from build123d import *

# Parameters (mm, degrees)
EXTRUDE_1_DEPTH     = 10
EXTRUDE_2_DEPTH     = 10
SKETCH_4_W          = 32
SKETCH_4_H          = 4
EXTRUDE_3_DEPTH     = 60
CUT_EXTRUDE_1_DEPTH = 30
SKETCH_6_W          = 12
SKETCH_6_H          = 10
EXTRUDE_4_DEPTH     = 40
SKETCH_7_W          = 10
SKETCH_7_H          = 5
EXTRUDE_5_DEPTH     = 100
SKETCH_9_R          = 5
EXTRUDE_7_DEPTH     = 5


with BuildPart() as part:
    # 草图1 → 凸台-拉伸1 (new body)
    with BuildSketch(Plane(origin=(0, 0, 0), x_dir=(1, 0, 0), z_dir=(0, 1, 0))):
        with BuildLine():
            Line((-50, 0), (-46, 0))
            ThreePointArc((-46, 0), (0, 46), (46, 0))
            Line((46, 0), (50, 0))
            ThreePointArc((50, 0), (0, 50), (-50, 0))
        make_face()
    extrude(amount=EXTRUDE_1_DEPTH)

    # 草图3 → 凸台-拉伸2 (add)
    with BuildSketch(Plane(origin=(0, 10, 0), x_dir=(1, 0, 0), z_dir=(0, 1, 0))):
        with BuildLine():
            Line((-50, 16), (-47.370877129, 16))
            ThreePointArc((-47.370877129, 16), (-36.689752119, 33.968545589), (-19.595917942, 46))
            Line((-19.595917942, 46), (-30, 46))
            Line((-30, 46), (-30, 50))
            Line((-30, 50), (30, 50))
            Line((30, 50), (30, 46))
            Line((30, 46), (19.595917942, 46))
            ThreePointArc((19.595917942, 46), (36.689752119, 33.968545589), (47.370877129, 16))
            Line((47.370877129, 16), (50, 16))
            Line((50, 16), (50, -16))
            Line((50, -16), (46, -16))
            Line((46, -16), (46, 0))
            ThreePointArc((46, 0), (0, 46), (-46, 0))
            Line((-46, 0), (-46, -16))
            Line((-46, -16), (-50, -16))
            Line((-50, -16), (-50, 16))
        make_face()
    extrude(amount=EXTRUDE_2_DEPTH)

    # 草图4 → 凸台-拉伸3 (add)
    with BuildSketch(Plane(origin=(0, 20, 0), x_dir=(1, 0, 0), z_dir=(0, 1, 0))):
        with Locations((0, 48)):
            Rectangle(SKETCH_4_W, SKETCH_4_H)
    extrude(amount=EXTRUDE_3_DEPTH)

    # 草图5 → 切除-拉伸1 (cut)
    with BuildSketch(Plane(origin=(0, 0, -50), x_dir=(-1, 0, 0), z_dir=(0, 0, -1))):
        with BuildLine():
            Line((-16, 64), (-16, 97.905328476))
            Line((-16, 97.905328476), (16, 97.905328476))
            Line((16, 97.905328476), (16, 64))
            ThreePointArc((16, 64), (0, 80), (-16, 64))
        make_face()
    extrude(amount=-CUT_EXTRUDE_1_DEPTH, mode=Mode.SUBTRACT)

    # 草图6 → 凸台-拉伸4 (add)
    with BuildSketch(Plane.ZY.offset(50)):
        with Locations((7, 15)):
            Rectangle(SKETCH_6_W, SKETCH_6_H)
    extrude(amount=EXTRUDE_4_DEPTH)

    # 草图7 → 凸台-拉伸5 (add)
    with BuildSketch(Plane(origin=(0, 20, 0), x_dir=(1, 0, 0), z_dir=(0, 1, 0))):
        with Locations((-85, -3.5)):
            Rectangle(SKETCH_7_W, SKETCH_7_H)
    extrude(amount=EXTRUDE_5_DEPTH)

    # 草图9 → 凸台-拉伸7 (add)
    with BuildSketch(Plane.XY.offset(6)):
        with Locations((-85, 120)):
            Circle(SKETCH_9_R)
    extrude(amount=-EXTRUDE_7_DEPTH)


solid = part.part
Verification items for the finished model (mm, model axes). A direction names the side the tool comes from. Give positions to 0.01 mm unless a question says otherwise; leave off trailing zeros. Order: outer loops, then holes, each group sorted by start corner. A loop starts at its lowest first (then second) coordinate and runs counter-clockwise, first axis right, second up. Notation, with made-up numbers: M 83,-13 L 113,-13 A12 ccw 113,-4 Z; hole C 21,7.25 d7. An arc over 180 degrees is marked long. Answer as a JSON object with one key per item and string values. Group by question number.
1) Scan lines: line 1 along Z through (x, y) = (4.5, 37); line 2 along X through (y, z) = (11.5, -40); line 3 along Y through (x, z) = (-48.5, -6). Record each from-to range of solid material in increasing order. Write a range as [from, to].
2) Mould release check, pull along Z, two halves, no side actions. Record for faces 1 (the face through (-25, 15, -46)), 2 (the face through (22, 10, -48)), 3 (the face through (-85, 73, 6)): released by +Z, released by -Z, zero draft, split by the parting line, or undercut.
3) Depth check by flat-ended pin: pin 1 Ø2 at (y, z) = (63.5, 2) entering from +X; pin 2 Ø5 at (x, y) = (-84.5, 89.5) entering from +Z; pin 3 Ø3 at (x, z) = (48.5, 4) entering from -Y. Enter the tip coordinate at first touch or a pass-through.
4) Access from +Z, -Z, +X, -X, +Y, -Y to the whole of each face (thin tool, end or side, straight path). Record for faces 4 (the face through (-50, 15, 15)), 5 (the face through (-21, 10, -48)), 6 (the face through (-50, 15, -7)), 7 (the face through (-80, 69, 4)), 8 (the face through (-46, 15, 8)).
5) Cross-section at B-B (y = 43.5). Enter the section's corners in (x, z).
6) Cross-section at C-C (x = -85). Enter the section's corners in (y, z), then the cut area to 3 significant figures.
7) Cross-section at A-A (z = -23). Enter the section's corners in (x, y).
8) Cross-section at D-D (z = -11). Enter the section's corners in (x, y) (3 decimals).
Result sheet:
{
 "1": {"line 1": "z = [-50, -46]", "line 2": "x = [-30, -22.72], [22.72, 30]", "line 3": "y = [0, 20]"},
 "2": {"face 1": "undercut", "face 2": "zero draft", "face 3": "released by +Z"},
 "3": {"pin 1": "stops at x = -80", "pin 2": "stops at z = 6", "pin 3": "stops at y = 10"},
 "4": {"face 4": "+Z, -X, +Y, -Y", "face 5": "-Z, -X, -Y", "face 6": "-Z, -X, +Y, -Y", "face 7": "+Z, -Z, +X, +Y", "face 8": "+Z, +Y, -Y"},
 "5": {"outline": "M -90,1 L -80,1 L -80,6 L -90,6 Z; M -16,-50 L 16,-50 L 16,-46 L -16,-46 Z"},
 "6": {"outline": "M 10,1 L 125,1 L 125,6 L 20,6 L 20,13 L 10,13 Z", "area": "645 mm2"},
 "7": {"outline": "M -44.4,0 L -39.84,0 L -39.84,20 L -44.4,20 Z; M 39.84,0 L 44.4,0 L 44.4,20 L 39.84,20 Z"},
 "8": {"outline": "M -50,10 L -48.775,10 L -48.775,0 L -44.665,0 L -44.665,20 L -50,20 Z; M 44.665,0 L 48.775,0 L 48.775,10 L 50,10 L 50,20 L 44.665,20 Z"}
}
